Work out the finished part from the listing and answer in its coordinate system (mm). A direction names the side the tool comes from. Give positions to 0.01 mm unless a question says otherwise; leave off trailing zeros. Write each loop counter-clockwise with the first axis right and the second up, starting at its lowest first coordinate (ties: lowest second). Pieces come first, ordered by that corner, then holes.
1) Find section A-A (y = 16). Determine the outline of the cut face in (x, z), plus the area to 3 significant figures.
2) Find section D-D (z = 15). Determine the outline of the cut face in (x, y), plus the area to 3 significant figures.
3) Find section C-C (y = 28.5). Determine the outline of the cut face in (x, z).
4) Find section B-B (x = 12.7). Determine the outline of the cut face in (y, z).
5) Determine the mould class of faces 5 (the face through (-72, 3, 24.96)), 6 (the face through (-6, 25.4, -19)) for opening direction X: pulls with the +X half, pulls with the -X half, needs draft (parallel to the pull), parting line crosses it, or undercut.
6) A tool of negligible diameter and unlimited length cuts with its end or side. For faces 1 (the face through (-72, 3, -15.04)), 2 (the face through (-26, 31.75, 5)), 3 (the face through (13, 3, 24.96)), 4 (the face through (-55.57, 31.84, 29.59)), from which of +Z, -Z, +X, -X, +Y, -Y can it reach the whole face along a straight path? Write none if from no direction.
7) Straight lines are drawn through the part: probe 1 along X at (y, z) = (25, -3); probe 2 along X at (y, z) = (6, 3); probe 3 along X at (y, z) = (2, -6.5). For each, find the intervals that lie inside material, in ascending order.
8) Given pin 1 Ø5 at (x, y) = (16.5, 3.5) entering from -Z; pin 2 Ø6 at (x, z) = (4, 26.5) entering from +Y; pin 3 Ø6 at (y, z) = (24.5, -13) entering from -X; pin 4 Ø5 at (x, z) = (-72.64, 17.34) entering from -Y, each flat-ended and moving along its own axis, determine where each tip first touches the part or whether it passes through.
```python
from build123d import *

# Parameters (mm, degrees)
SKETCH1_W           = 59.944
SKETCH1_H           = 59.944
BOSS_EXTRUDE1_DEPTH = 38.1
SKETCH2_W           = 34.544
SKETCH2_H           = 31.75
CUT_EXTRUDE1_DEPTH  = 93.941789697
SKETCH3_R           = 3.175
CUT_EXTRUDE2_DEPTH  = 80.152691578
SKETCH4_W           = 40
SKETCH4_H           = 6.35
BOSS_EXTRUDE2_DEPTH = 25.4
SKETCH5_W           = 40
SKETCH5_H           = 6.35
BOSS_EXTRUDE3_DEPTH = 25.4
SKETCH6_R           = 4
CUT_EXTRUDE3_DEPTH  = 98.529053538
SKETCH7_R           = 2.286
CUT_EXTRUDE4_DEPTH  = 12.7


with BuildPart() as part:
    # Sketch1 → Boss-Extrude1 (new body)
    with BuildSketch(Plane(origin=(0, 0, 0), x_dir=(1, 0, 0), z_dir=(0, 1, 0))):
        with Locations((-29.972, -4.96015493)):
            Rectangle(SKETCH1_W, SKETCH1_H)
    extrude(amount=BOSS_EXTRUDE1_DEPTH)

    # Sketch2 → Cut-Extrude1 (cut, through all)
    with BuildSketch(Plane.XY.offset(34.93215493)):
        with Locations((-29.972, 15.875)):
            Rectangle(SKETCH2_W, SKETCH2_H)
    extrude(amount=-CUT_EXTRUDE1_DEPTH, mode=Mode.SUBTRACT)

    # Sketch3 → Cut-Extrude2 (cut, through all)
    with BuildSketch(Plane(origin=(0, 38.1, 0), x_dir=(1, 0, 0), z_dir=(0, 1, 0))):
        with Locations(Location((-29.972, -4.96015493, 0), (0, 0, 270))):
            Circle(SKETCH3_R)
    extrude(amount=-CUT_EXTRUDE2_DEPTH, mode=Mode.SUBTRACT)

    # Sketch4 → Boss-Extrude2 (add)
    with BuildSketch(Plane(origin=(0, 0, 0), x_dir=(0, 0, -1), z_dir=(1, 0, 0))):
        with Locations((-4.960154808, 3.175)):
            Rectangle(SKETCH4_W, SKETCH4_H)
    extrude(amount=BOSS_EXTRUDE2_DEPTH)

    # Sketch5 → Boss-Extrude3 (add)
    with BuildSketch(Plane.ZY.offset(59.944)):
        with Locations((4.960154808, 3.175)):
            Rectangle(SKETCH5_W, SKETCH5_H)
    extrude(amount=BOSS_EXTRUDE3_DEPTH)

    # Sketch6 → Cut-Extrude3 (cut, through all)
    with BuildSketch(Plane(origin=(0, 6.35, 0), x_dir=(1, 0, 0), z_dir=(0, 1, 0))):
        with Locations(Location((-72.644, 7.419845192, 0), (0, 0, 270))):
            Circle(SKETCH6_R)
        with Locations(Location((-72.644, -17.340154808, 0), (0, 0, 270))):
            Circle(SKETCH6_R)
        with Locations(Location((12.7, 7.419845192, 0), (0, 0, 270))):
            Circle(SKETCH6_R)
        with Locations(Location((12.7, -17.340154808, 0), (0, 0, 270))):
            Circle(SKETCH6_R)
    extrude(amount=-CUT_EXTRUDE3_DEPTH, mode=Mode.SUBTRACT)

    # Sketch7 → Cut-Extrude4 (cut)
    with BuildSketch(Plane(origin=(0, 38.1, 0), x_dir=(1, 0, 0), z_dir=(0, 1, 0))):
        with Locations(Location((-53.5432, 18.61104507, 0), (0, 0, 270))):
            Circle(SKETCH7_R)
        with Locations(Location((-6.4008, -28.53135493, 0), (0, 0, 270))):
            Circle(SKETCH7_R)
        with Locations(Location((-53.5432, -28.53135493, 0), (0, 0, 270))):
            Circle(SKETCH7_R)
        with Locations(Location((-6.4008, 18.61104507, 0), (0, 0, 270))):
            Circle(SKETCH7_R)
    extrude(amount=-CUT_EXTRUDE4_DEPTH, mode=Mode.SUBTRACT)


solid = part.part
```
Results:
1. outline: (-59.94, -25.01) - (-47.24, -25.01) - (-47.24, 34.93) - (-59.94, 34.93) - close; (-12.7, -25.01) - (0, -25.01) - (0, 34.93) - (-12.7, 34.93) - close
1. area: 1,520 mm2
2. outline: (-85.34, 0) - (-75.89, 0) - (-75.89, 6.35) - (-85.34, 6.35) - close; (-69.4, 0) - (-47.24, 0) - (-47.24, 31.75) - (-12.7, 31.75) - (-12.7, 0) - (9.46, 0) - (9.46, 6.35) - (0, 6.35) - (0, 38.1) - (-59.94, 38.1) - (-59.94, 6.35) - (-69.4, 6.35) - close; (15.94, 0) - (25.4, 0) - (25.4, 6.35) - (15.94, 6.35) - close
2. area: 1,430 mm2
3. outline: (-59.94, -25.01) - (-47.24, -25.01) - (-47.24, 34.93) - (-59.94, 34.93) - close; (-12.7, -25.01) - (0, -25.01) - (0, 34.93) - (-12.7, 34.93) - close; hole circle Ø4.57 at (-53.54, -18.61); hole circle Ø4.57 at (-53.54, 28.53); hole circle Ø4.57 at (-6.4, -18.61); hole circle Ø4.57 at (-6.4, 28.53)
4. outline: (0, -15.04) - (6.35, -15.04) - (6.35, -11.42) - (0, -11.42) - close; (0, -3.42) - (6.35, -3.42) - (6.35, 13.34) - (0, 13.34) - close; (0, 21.34) - (6.35, 21.34) - (6.35, 24.96) - (0, 24.96) - close
5. face 5: needs draft
5. face 6: undercut
6. face 1: -Z, -X, +Y, -Y
6. face 2: +Z, -Z, -Y
6. face 3: +Z, +X, +Y, -Y
6. face 4: +Y
7. probe 1: x = -59.94 to -47.24, -12.7 to 0
7. probe 2: x = -85.34 to -47.24, -12.7 to 25.4
7. probe 3: x = -85.34 to -76.54, -68.75 to -47.24, -12.7 to 8.81, 16.59 to 25.4
8. pin 1: stops at z = -15.04
8. pin 2: stops at y = 6.35
8. pin 3: stops at x = -59.94
8. pin 4: passes through
